The drawing under review shows one solid part. Ordinate dimensions are in mm from its lowest x, y, z. A direction names the side the tool comes from. Coordinates: 2 decimals unless noted, no trailing zeros. Order: outer loops, then holes, each group sorted by start corner. A loop starts at its lowest first (then second) coordinate and runs counter-clockwise, first axis right, second up.
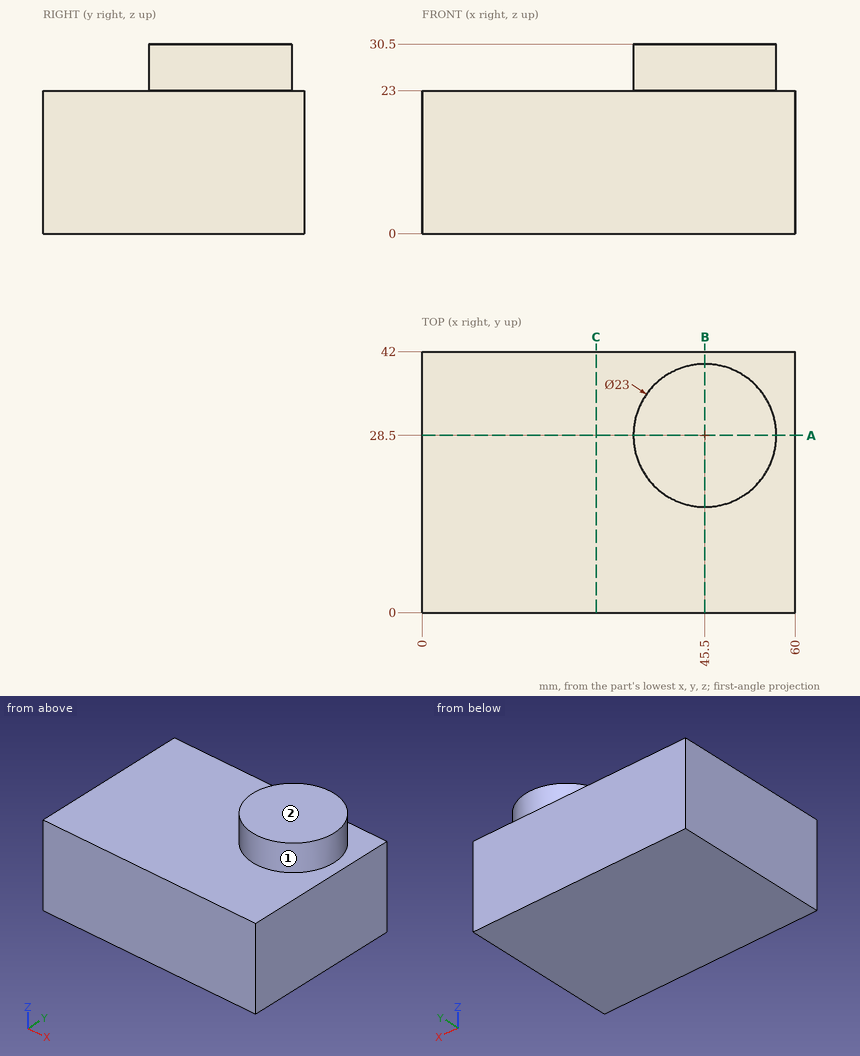
1. To check wall thickness, follow L1, parallel to Z at x = 23, y = 3; L2, parallel to X at y = 21.5, z = 24.5; L3, parallel to X at y = 19.5, z = 24. State the ranges of each line that lie inside material, in increasing order.
Answer below:
L1: z = 0 to 23
L2: x = 36.38 to 54.62
L3: x = 38.34 to 52.66
2. Take a section at A-A, the plane y = 28.5. Give the boundary of the cut face in (x, z).
Answer below:
outline: (0, 0) - (60, 0) - (60, 23) - (57, 23) - (57, 30.5) - (34, 30.5) - (34, 23) - (0, 23) - close
3. Take a section at C-C, the plane x = 28. Give the boundary of the cut face in (y, z), plus the area to 3 significant figures.
Answer below:
outline: (0, 0) - (42, 0) - (42, 23) - (0, 23) - close
area: 966 mm2
4. Take a section at B-B, the plane x = 45.5. Give the boundary of the cut face in (y, z).
Answer below:
outline: (0, 0) - (42, 0) - (42, 23) - (40, 23) - (40, 30.5) - (17, 30.5) - (17, 23) - (0, 23) - close
5. Clearance check with a flat-ended pin moving along its axis: pin 1 Ø3 at (x, y) = (6, 33) entering from +Z. State where the tip first meets the part, or that it passes through.
Answer below:
pin 1: stops at z = 23
6. Machinability: for the marked faces 1 and 2, which of the approach directions +Z, -Z, +X, -X, +Y, -Y give a long, thin tool a straight path to every point of the face, cutting with its end or side? Answer none if there is none.
Answer below:
face 1: +Z
face 2: +Z, +X, -X, +Y, -Y
